Design review of the part built by this model. Coordinates are the model's own, in mm. A direction names the side the tool comes from. Coordinates: 2 decimals unless noted, no trailing zeros. Order: outer loops, then holes, each group sorted by start corner. A loop starts at its lowest first (then second) coordinate and runs counter-clockwise, first axis right, second up.
from build123d import *

# Parameters (mm, degrees)
SKETCH_1_W          = 42
SKETCH_1_H          = 45
SKETCH_1_R          = 12.5
EXTRUDE_1_DEPTH     = 12
SKETCH_2_R          = 3
CUT_EXTRUDE_2_DEPTH = 10


with BuildPart() as part:
    # 草图1 → 凸台-拉伸1 (new body)
    with BuildSketch(Plane.XY):
        Rectangle(SKETCH_1_W, SKETCH_1_H)
        Circle(SKETCH_1_R, mode=Mode.SUBTRACT)
        with BuildLine():
            Line((-14, 17), (-14, 14))
            ThreePointArc((-14, 14), (-15.5, 12.5), (-17, 14))
            Line((-17, 14), (-17, 17))
            ThreePointArc((-17, 17), (-15.5, 18.5), (-14, 17))
        make_face(mode=Mode.SUBTRACT)
        with BuildLine():
            Line((14, 17), (14, 14))
            ThreePointArc((14, 14), (15.5, 12.5), (17, 14))
            Line((17, 14), (17, 17))
            ThreePointArc((17, 17), (15.5, 18.5), (14, 17))
        make_face(mode=Mode.SUBTRACT)
        with BuildLine():
            Line((14, -17), (14, -14))
            ThreePointArc((14, -14), (15.5, -12.5), (17, -14))
            Line((17, -14), (17, -17))
            ThreePointArc((17, -17), (15.5, -18.5), (14, -17))
        make_face(mode=Mode.SUBTRACT)
        with BuildLine():
            Line((-14, -17), (-14, -14))
            ThreePointArc((-14, -14), (-15.5, -12.5), (-17, -14))
            Line((-17, -14), (-17, -17))
            ThreePointArc((-17, -17), (-15.5, -18.5), (-14, -17))
        make_face(mode=Mode.SUBTRACT)
    extrude(amount=EXTRUDE_1_DEPTH)

    # 草图2 → 切除-拉伸2 (cut)
    with BuildSketch(Plane(origin=(0, 22.5, 0), x_dir=(1, 0, 0), z_dir=(0, 1, 0))):
        with Locations(Location((-9, -6, 0), (0, 0, 180))):
            Circle(SKETCH_2_R)
        with Locations(Location((9, -6, 0), (0, 0, 180))):
            Circle(SKETCH_2_R)
    extrude(amount=-CUT_EXTRUDE_2_DEPTH, mode=Mode.SUBTRACT)


solid = part.part
1. Add section C-C (x = 4). Give the boundary of the cut face in (y, z).
2. Add section B-B (x = 15.5). Give the boundary of the cut face in (y, z), and give its area (3 significant figures).
3. To check wall thickness, follow line 1 (Y direction, x = -15.5, z = 10.5); line 2 (Z direction, x = -9, y = 16); line 3 (Y direction, x = 0, z = 6.5). State the ranges of each line that lie inside material, in increasing order.
4. Mouldability with a two-part tool opening along Y and no side actions: class faces 1 (the flat face through (21, 0, 6)), 2 (the cylindrical face through (-15.5, 18.5, 5.9)), 3 (the flat face through (9, 12.5, 6)) as pulls with the +Y half, pulls with the -Y half, needs draft (parallel to the pull), parting line crosses it, or undercut.
5. Insertion check: pin 1 (5.5 mm diameter, centred on x = -9, z = 6, fed in from +Y). The pin has a flat end and moves straight along its axis. Give the tip position at first contact, or say it passes through.
6. Add section A-A (y = 0). Give the boundary of the cut face in (x, z), and give its area (3 significant figures).
7. Add section D-D (z = 6.75). State how many separate pieces and enclosed holes the cut face has, and give its area (3 significant figures).
8. For faces 4 (the flat face through (-17, -15, 6)), 5 (the cylindrical face through (9.65, 17.57, 3.07)), 6 (the flat face through (9, 10, 0)), list the 3-axis set-ups (+Z, -Z, +X, -X, +Y, -Y) from which the entire face can be reached by the end or side of a thin tool; tool diameter is ignored.
Solution:
1. outline: (-22.5, 0) - (-11.84, 0) - (-11.84, 12) - (-22.5, 12) - close; (11.84, 0) - (22.5, 0) - (22.5, 12) - (11.84, 12) - close
2. outline: (-22.5, 0) - (-18.5, 0) - (-18.5, 12) - (-22.5, 12) - close; (-12.5, 0) - (12.5, 0) - (12.5, 12) - (-12.5, 12) - close; (18.5, 0) - (22.5, 0) - (22.5, 12) - (18.5, 12) - close
2. area: 396 mm2
3. line 1: y = -22.5 to -18.5, -12.5 to 12.5, 18.5 to 22.5
3. line 2: z = 0 to 3, 9 to 12
3. line 3: y = -22.5 to -12.5, 12.5 to 22.5
4. face 1: needs draft
4. face 2: undercut
4. face 3: pulls with the +Y half
5. pin 1: stops at y = 12.5
6. outline: (-21, 0) - (-12.5, 0) - (-12.5, 12) - (-21, 12) - close; (12.5, 0) - (21, 0) - (21, 12) - (12.5, 12) - close
6. area: 204 mm2
7. separate pieces: 1
7. enclosed holes: 5
7. area: 1,220 mm2
8. face 4: +Z, -Z
8. face 5: +Y
8. face 6: -Z, +X, -X, +Y, -Y
